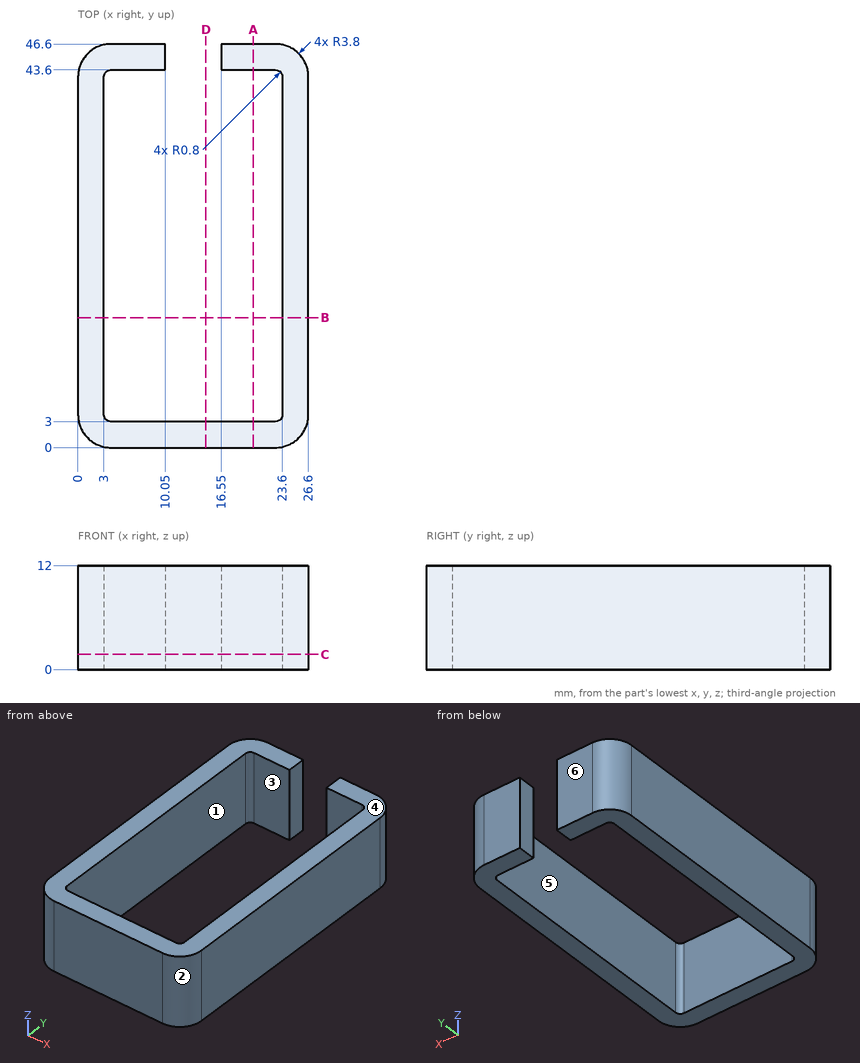
The drawing under review shows one solid part. Ordinate dimensions are in mm from its lowest x, y, z. A direction names the side the tool comes from. Coordinates: 2 decimals unless noted, no trailing zeros. Write each loop counter-clockwise with the first axis right and the second up, starting at its lowest first coordinate (ties: lowest second). Pieces come first, ordered by that corner, then holes. Notation, with made-up numbers: (77.5, 86) - (119.5, 86) arc R33 ccw to (119.5, 120) - close; hole circle Ø1 at (27, 72.25). An arc over 180 degrees is marked (long way). Put each result on its own line as item: value.
1. Add section C-C, the plane z = 1.75. Give the boundary of the cut face in (x, y), then the cut area to 3 significant figures.
Values found:
outline: (0, 3.8) arc R3.8 ccw to (3.8, 0) - (22.8, 0) arc R3.8 ccw to (26.6, 3.8) - (26.6, 42.8) arc R3.8 ccw to (22.8, 46.6) - (16.55, 46.6) - (16.55, 43.6) - (22.8, 43.6) arc R0.8 cw to (23.6, 42.8) - (23.6, 3.8) arc R0.8 cw to (22.8, 3) - (3.8, 3) arc R0.8 cw to (3, 3.8) - (3, 42.8) arc R0.8 cw to (3.8, 43.6) - (10.05, 43.6) - (10.05, 46.6) - (3.8, 46.6) arc R3.8 ccw to (0, 42.8) - close
area: 372 mm²
2. Add section D-D, the plane x = 14.75. Give the boundary of the cut face in (y, z), then the cut area to 3 significant figures.
Values found:
outline: (0, 0) - (3, 0) - (3, 12) - (0, 12) - close
area: 36.0 mm²
3. Mouldability with a two-part tool opening along Y and no side actions: class the marked faces 3, 4, 5 and 6 as released by +Y, released by -Y, zero draft, split by the parting line, or undercut.
Values found:
face 3: undercut
face 4: zero draft
face 5: undercut
face 6: released by +Y
4. For pin 1 (2 mm diameter, centred on x = 13, z = 8, fed in from +Y); pin 2 (2.5 mm diameter, centred on y = 45, z = 4, fed in from +X); pin 3 (1.5 mm diameter, centred on x = 23, z = 6.5, fed in from +Y); pin 4 (2.5 mm diameter, centred on y = 45, z = 6.5, fed in from -X), all flat-tipped, find the tip position at first contact; note any pin that passes through.
Values found:
pin 1: y = 3
pin 2: x = 26.48
pin 3: y = 46.6
pin 4: x = 0.12
5. Add section B-B, the plane y = 15. Give the boundary of the cut face in (x, z), then the cut area to 3 significant figures.
Values found:
outline: (0, 0) - (3, 0) - (3, 12) - (0, 12) - close; (23.6, 0) - (26.6, 0) - (26.6, 12) - (23.6, 12) - close
area: 72.0 mm²
6. Machinability: for the marked faces 1 and 2, which of the approach directions +Z, -Z, +X, -X, +Y, -Y give a long, thin tool a straight path to every point of the face, cutting with its end or side? Answer none if there is none.
Values found:
face 1: +Z, -Z
face 2: +Z, -Z, +X, -Y
7. Wall thickness on probe 1 along Y at (x, z) = (7.5, 1.25); probe 2 along X at (y, z) = (11.5, 8.5); probe 3 along Y at (x, z) = (14.75, 3.75): over which ranges is each line inside the solid? List them lowest first.
Values found:
probe 1: 0 to 3, 43.6 to 46.6
probe 2: 0 to 3, 23.6 to 26.6
probe 3: 0 to 3
8. Add section A-A, the plane x = 20.25. Give the boundary of the cut face in (y, z).
Values found:
outline: (0, 0) - (3, 0) - (3, 12) - (0, 12) - close; (43.6, 0) - (46.6, 0) - (46.6, 12) - (43.6, 12) - close
